Autodesk Inventor part; units mm, degrees
ref_plane "Work Plane11" through (7.5, 24, 68.0467) normal (0, 0, -1) x (-1, 0, 0)
ref_plane "YZ Plane" through (0, 0, 0) normal (1, 0, 0) x (0, 1, 0)
ref_plane "XZ Plane" through (0, 0, 0) normal (0, 1, 0) x (-1, 0, 0)
sketch "Sketch1" plane through (0, 0, 0) normal (0, 1, 0) x (-1, 0, 0)
  arc A0 (-8.5938, 6.8664) -> (8.5938, 6.8664) centre (0, 0) ccw
  line L0 (-7.5, 9.9875) -> (-7.5, 18.0467)
  line L1 (7.5, 18.0467) -> (7.5, 9.9875)
  line L2 (7.5, 18.0467) -> (-7.5, 18.0467)
  arc A1 (7.5, 9.9875) -> (8.5938, 6.8664) centre (12.5, 9.9875) ccw
  arc A2 (-8.5938, 6.8664) -> (-7.5, 9.9875) centre (-12.5, 9.9875) ccw
  point P0 (7.5, 8.0467)
  point P1 (-7.5, 8.0467)
  point P2 (0, 8.0467)
  point P3 (0, 18.0467)
  dimension "d0" = 22
  dimension "d109" = 5
  dimension "d129" = 15
  dimension "d131" = 10
extrude "Extrusion1" add sketch "Sketch1" against normal blind 12
sketch "Sketch22" plane through (-7.5, 0, 18.0467) normal (0, 0, 1) x (1, 0, 0)
  line L0 (0, 0) -> (0, -12)
  line L1 (15, -12) -> (0, -12)
  line L2 (0, 0) -> (15, 0)
  line L3 (15, 0) -> (15, -12)
  line L4 (15, -12) -> (0, -12)
  line L5 (0, -12) -> (0, 0)
  point P0 (7.5, 0)
sketch "Sketch23" plane through (0, 0, 0) normal (1, 0, 0) x (0, 1, 0)
  line L0 (0, 18.0467) -> (-12, 18.0467)
  line L1 (-6, 18.0467) -> (-6, 38.0467)
  line L2 (24, 68.0467) -> (155.224, 68.0467)
  arc A0 (24, 68.0467) -> (-6, 38.0467) centre (24, 38.0467) ccw
  point P0 (0, 0)
  point P1 (-6, 68.0467)
  dimension "d110" = 50
  dimension "d111" = 161.224
  dimension "d112" = 90
  dimension "d113" = 30
sweep "Sweep2" add profiles "Sketch22" path "Sketch23" path curves L1 A0 L2
ref_plane "Work Plane11" through (7.5, 24, 68.0467) normal (0, 0, -1) x (-1, 0, 0)
sketch "Sketch24" plane through (7.5, 24, 68.0467) normal (0, 0, -1) x (-1, 0, 0)
  line L0 (0, 131.224) -> (15, 131.224)
  line L1 (0, 131.224) -> (15, 131.224)
  line L2 (0, 131.224) -> (0, 135.1772)
  line L3 (15, 131.224) -> (15, 135.1772)
  arc A0 (15, 135.1772) -> (0, 135.1772) centre (7.5, 143.224) ccw
  point P0 (7.5, -24)
  point P1 (7.5, 131.224)
  point P2 (7.5, 131.224)
  dimension "d142" = 22
  dimension "d143" = 12
extrude "Extrusion17" add sketch "Sketch24" along normal mid plane 12
sketch "Sketch25" plane through (-7.5, 24, 74.0467) normal (0, 0, 1) x (1, 0, 0)
  circle A0 centre (7.5, 143.224) radius 2.5
  arc A1 (15, 135.1772) -> (0, 135.1772) centre (7.5, 143.224) ccw
  point P0 (7.5, -24)
  point P1 (22.3607, 44.2893)
  point P2 (7.3607, 44.2893)
  dimension "d123" = 5
extrude "Extrusion18" cut sketch "Sketch25" against normal through all
sketch "Sketch27" plane through (0, 0, 0) normal (0, 1, 0) x (1, 0, 0)
  arc A0 (8.5938, -6.8664) -> (-8.5938, -6.8664) centre (0, 0) ccw
  circle A1 centre (0, 0) radius 2.4
  dimension "d136" = 4.8
extrude "Extrusion20" add sketch "Sketch27" against normal blind 26
sketch "Sketch29" plane through (7.5, 24, 62.0467) normal (0, 0, -1) x (-1, 0, 0)
  circle A0 centre (7.5, 143.224) radius 2.5
  circle A1 centre (7.5, 143.224) radius 8.1
  point P0 (7.5, -24)
  dimension "d144" = 16.2
extrude "Extrusion22" cut sketch "Sketch29" against normal blind 5
mirror "Mirror2" about plane through (7.5, 24, 68.0467) normal (0, 0, -1) of "Extrusion22"
sketch "Sketch30" plane through (0, 0, 0) normal (0, 1, 0) x (1, 0, 0)
  line L0 (3.1754, 0) -> (1.5877, -2.75)
  line L1 (1.5877, -2.75) -> (-1.5877, -2.75)
  line L2 (-1.5877, -2.75) -> (-3.1754, 0)
  line L3 (-3.1754, 0) -> (-1.5877, 2.75)
  line L4 (-1.5877, 2.75) -> (1.5877, 2.75)
  line L5 (1.5877, 2.75) -> (3.1754, 0)
  point P0 (0, 0)
  point P1 (0, 0)
  point P2 (0, 0)
  dimension "d148" = 5.5
extrude "Extrusion23" cut sketch "Sketch30" against normal blind 3
sketch "Sketch31" plane through (0, -3, 0) normal (0, 1, 0) x (1, 0, 0)
  circle A0 centre (0, 0) radius 1.6
  dimension "d151" = 3.2
extrude "Extrusion24" cut sketch "Sketch31" against normal through all
properties part number "distal_link_1"
The model under review builds one solid part; all positions refer to its coordinate system, in mm. A direction names the side the tool comes from. Round coordinates to 2 decimals unless told otherwise and drop trailing zeros. Loops run counter-clockwise (first coordinate to the right, second up) from the corner with the lowest first, then second, coordinate; pieces in that order, holes last. Notation, with made-up numbers: M 63.5,60 L 85.5,60 A28 cw 85.5,82 Z; hole C 2,27 d10. An arc over 180 degrees is marked long. Answer as a JSON object with one key per item and string values.
Item 1: The part is to be moulded in two halves that separate along X. For faces 5 (the face through (0, -26, 2)), 6 (the face through (7.5, 55, 63)), 7 (the face through (0.368, 178.218, 68.131)), 8 (the face through (1.756, 159.317, 64.512)), say which applies: +X half, -X half, draft (parallel to the pull), parting line (faces both ways), or undercut.
Check sheet entries:
{"face 5": "draft", "face 6": "+X half", "face 7": "parting line", "face 8": "undercut"}
Item 2: For line 1 along X through (y, z) = (-9, 0); line 2 along X through (y, z) = (35, 70.5); line 3 along Z through (x, y) = (-6, 135.5), list the stretches that pass through material, from the lowest coordinate up.
Check sheet entries:
{"line 1": "-11 to -1.6, 1.6 to 11", "line 2": "-7.5 to 7.5", "line 3": "62.05 to 74.05"}
Item 3: We need section B-B, the plane z = 35. State the section outline as (x, y) points.
Check sheet entries:
{"outline": "M -7.5,-12 L 7.5,-12 L 7.5,0 L -7.5,0 Z"}
Item 4: Tool access review of faces 1 (the face through (1.4, -3, -1.3)), 2 (the face through (0, 0, 13)), 3 (the face through (-7.5, 61, 64)), 4 (the face through (2, 169, 69.047)): name each direction out of +Z, -Z, +X, -X, +Y, -Y from which nothing blocks a thin tool from reaching the whole face with its end or side.
Check sheet entries:
{"face 1": "+Y", "face 2": "-Z, +X, -X, +Y", "face 3": "+Z, -X, -Y", "face 4": "+Z"}
Item 5: Clearance check with flat-ended pins moving along their axes: P1, Ø13, axis at x = 0, y = 167.224, coming from the +Z side; P2, Ø11, axis at x = 1, z = 2, coming from the +Y side; P3, Ø2.5, axis at x = 0.5, y = -2, coming from the +Z side; P4, Ø1.9, axis at x = 0, z = 0, coming from the -Y side. State where each tip first meets the part, or that it passes through.
Check sheet entries:
{"P1": "z = 69.05", "P2": "y = 0", "P3": "z = 64.19", "P4": "through"}
Item 6: We need section A-A, the plane y = 87. State the section outline as (x, z) points.
Check sheet entries:
{"outline": "M -7.5,62.05 L 7.5,62.05 L 7.5,74.05 L -7.5,74.05 Z"}
